```python
from build123d import *

# Parameters (mm, degrees)
SKETCH1_W           = 40
SKETCH1_H           = 40
BOSS_EXTRUDE1_DEPTH = 30
SHELL1_T            = -3
SKETCH2_W           = 40
SKETCH2_H           = 40
BOSS_EXTRUDE2_DEPTH = 3
SKETCH3_W           = 30
SKETCH3_H           = 9
CUT_EXTRUDE1_DEPTH  = 3
FILLET1_R           = 1


with BuildPart() as part:
    # Sketch1 → Boss-Extrude1 (new body)
    with BuildSketch(Plane(origin=(0, 0, 0), x_dir=(1, 0, 0), z_dir=(0, 1, 0))):
        Rectangle(SKETCH1_W, SKETCH1_H)
    extrude(amount=BOSS_EXTRUDE1_DEPTH)

    # Shell1
    shell1_openings = [part.faces().sort_by_distance(p)[0] for p in [
        (0, 30, 0),
    ]]
    offset(amount=SHELL1_T, openings=shell1_openings, kind=Kind.INTERSECTION)

    # Sketch2 → Boss-Extrude2 (add)
    with BuildSketch(Plane(origin=(0, 30, 0), x_dir=(1, 0, 0), z_dir=(0, 1, 0))):
        Rectangle(SKETCH2_W, SKETCH2_H)
    extrude(amount=BOSS_EXTRUDE2_DEPTH)

    # Sketch3 → Cut-Extrude1 (cut)
    with BuildSketch(Plane(origin=(0, 33, 0), x_dir=(1, 0, 0), z_dir=(0, 1, 0))):
        with Locations((0, -10.5)):
            Rectangle(SKETCH3_W, SKETCH3_H)
        with Locations((0, 10.5)):
            Rectangle(SKETCH3_W, SKETCH3_H)
    extrude(amount=-CUT_EXTRUDE1_DEPTH, mode=Mode.SUBTRACT)

    # Fillet1
    fillet1_edges = [part.edges().sort_by_distance(p)[0] for p in [
        (-20, 33, 0),
        (0, 33, 20),
        (20, 33, 0),
        (0, 33, -20),
        (0, 0, 20),
        (-15, 33, 10.5),
        (0, 33, 15),
        (15, 33, 10.5),
        (0, 33, 6),
        (-20, 0, 0),
        (-15, 33, -10.5),
        (0, 33, -6),
        (15, 33, -10.5),
        (0, 0, -20),
        (0, 33, -15),
        (20, 0, 0),
        (20, 16.5, 20),
        (-20, 16.5, 20),
        (-20, 16.5, -20),
        (20, 16.5, -20),
    ]]
    fillet(fillet1_edges, radius=FILLET1_R)


solid = part.part
```
Check sheet for the modelled part. Datum: model origin and axes. Units: mm. A direction names the side the tool comes from. Round coordinates to 2 decimals unless told otherwise and drop trailing zeros. Order: outer loops, then holes, each group sorted by start corner. A loop starts at its lowest first (then second) coordinate and runs counter-clockwise, first axis right, second up. Notation, with made-up numbers: (50, -7.5) - (78, -7.5) arc R32 cw to (78, 29.5) - close; hole circle Ø4 at (77, 6). An arc over 180 degrees is marked (long way). Write item = value, one per line.
Q1. Tool access check on faces 1 (the face through (-15, 31, -10)), 2 (the face through (0.266, 32.715, 19.699)), 3 (the face through (0, 16, 17)). Record the directions out of +Z, -Z, +X, -X, +Y, -Y that give a thin tool (end or side, any length) a straight path to the whole face; none if there is none.
Computed:
face_1 = +Y
face_2 = +Z, +X, -X, +Y
face_3 = none
Q2. Thickness scan on line 1 along X through (y, z) = (18.5, 4); line 2 along Y through (x, z) = (-15, -16). Record the ranges inside material, lowest first.
Computed:
line_1 = -20 to -17, 17 to 20
line_2 = 0 to 3, 30 to 33
Q3. Section check A-A (y = 27). Record the boundary of the cut face in (x, z), and give its area (3 significant figures).
Computed:
outline = (-20, -19) arc R1 ccw to (-19, -20) - (19, -20) arc R1 ccw to (20, -19) - (20, 19) arc R1 ccw to (19, 20) - (-19, 20) arc R1 ccw to (-20, 19) - close; hole (-17, -17) - (17, -17) - (17, 17) - (-17, 17) - close
area = 443 mm^2
Q4. Draft check along Z on faces 4 (the face through (0.266, 0.285, 19.699)), 5 (the face through (19.699, 0.285, -0.266)), 6 (the face through (-15, 31, 11)). Enter one of: pulls with the +Z half, pulls with the -Z half, needs draft (parallel to the pull), parting line crosses it, or undercut.
Computed:
face_4 = pulls with the +Z half
face_5 = needs draft
face_6 = undercut
Q5. Go/stop test with a flat-tipped pin: pin 1 (10 mm diameter, centred on x = 0.5, z = 7, fed in from +Y). Record where the tip stops, or that it passes through.
Computed:
pin_1 = 33
Q6. Section check B-B (x = 13.5). Record the boundary of the cut face in (y, z), and give its area (3 significant figures).
Computed:
outline = (0, -19) arc R1 ccw to (1, -20) - (32, -20) arc R1 ccw to (33, -19) - (33, -16) arc R1 ccw to (32, -15) - (30, -15) - (30, -17) - (3, -17) - (3, 17) - (30, 17) - (30, 15) - (32, 15) arc R1 ccw to (33, 16) - (33, 19) arc R1 ccw to (32, 20) - (1, 20) arc R1 ccw to (0, 19) - close; (30, -6) - (32, -6) arc R1 ccw to (33, -5) - (33, 5) arc R1 ccw to (32, 6) - (30, 6) - close
area = 346 mm^2
Q7. Section check D-D (z = 8.5). Record the boundary of the cut face in (x, y).
Computed:
outline = (-20, 1) arc R1 ccw to (-19, 0) - (19, 0) arc R1 ccw to (20, 1) - (20, 32) arc R1 ccw to (19, 33) - (16, 33) arc R1 ccw to (15, 32) - (15, 30) - (17, 30) - (17, 3) - (-17, 3) - (-17, 30) - (-15, 30) - (-15, 32) arc R1 ccw to (-16, 33) - (-19, 33) arc R1 ccw to (-20, 32) - close
Q8. Section check C-C (z = -2.5). Record the boundary of the cut face in (x, y).
Computed:
outline = (-20, 1) arc R1 ccw to (-19, 0) - (19, 0) arc R1 ccw to (20, 1) - (20, 32) arc R1 ccw to (19, 33) - (-19, 33) arc R1 ccw to (-20, 32) - close; hole (-17, 3) - (17, 3) - (17, 30) - (-17, 30) - close
